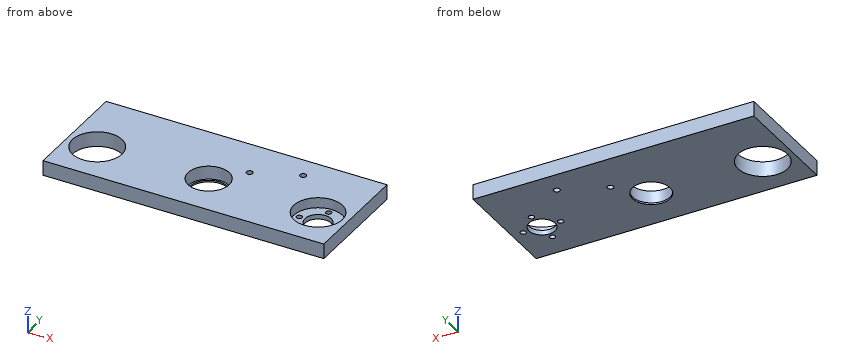
from build123d import *

# Parameters (mm, degrees)
ESQUISSE1_W                  = 150
ESQUISSE1_H                  = 60
BOSS_EXTRU_1_DEPTH           = 8
ENL_V_MAT_EXTRU_1_DEPTH      = 162.752897965
ENL_V_MAT_EXTRU_1_DEPTH_BACK = 7.1
ESQUISSE2_R                  = 11
ESQUISSE3_R                  = 10
ENL_V_MAT_EXTRU_2_DEPTH      = 162.710883987
ESQUISSE4_R                  = 7
ENL_V_MAT_EXTRU_3_DEPTH      = 162.752897965
ESQUISSE5_R                  = 13
ENL_V_MAT_EXTRU_4_DEPTH      = 5.5
ENL_V_MAT_EXTRU_5_DEPTH      = 162.752897965
ENL_V_MAT_EXTRU_5_DEPTH_BACK = 162.752897965
ESQUISSE6_R                  = 13.25
ENL_V_MAT_EXTRU_6_DEPTH      = 162.752897965
ENL_V_MAT_EXTRU_6_DEPTH_BACK = 162.752897965
ESQUISSE7_R                  = 1.65
ENL_V_MAT_EXTRU_7_DEPTH      = 162.648538503
ENL_V_MAT_EXTRU_7_DEPTH_BACK = 162.648538503
ESQUISSE8_R                  = 1.5


with BuildPart() as part:
    # Esquisse1 → Boss.-Extru.1 (new body)
    with BuildSketch(Plane.XY):
        with Locations((75, 30)):
            Rectangle(ESQUISSE1_W, ESQUISSE1_H)
    extrude(amount=BOSS_EXTRU_1_DEPTH)

    # Esquisse2 → Enlèv. mat.-Extru.1 (cut, two sides: drawn at the far end of the back side and taken through both)
    with BuildSketch(Plane.XY.offset(8).offset(-ENL_V_MAT_EXTRU_1_DEPTH_BACK)):
        with Locations(Location((75, 24, 0), (0, 0, 180))):
            Circle(ESQUISSE2_R)
    extrude(amount=ENL_V_MAT_EXTRU_1_DEPTH + ENL_V_MAT_EXTRU_1_DEPTH_BACK, mode=Mode.SUBTRACT)

    # Esquisse3 → Enlèv. mat.-Extru.2 (cut, through all)
    with BuildSketch(Plane.XY.offset(0.9)):
        with Locations((75, 24)):
            Circle(ESQUISSE3_R)
    extrude(amount=-ENL_V_MAT_EXTRU_2_DEPTH, mode=Mode.SUBTRACT)

    # Esquisse4 → Enlèv. mat.-Extru.3 (cut, through all)
    with BuildSketch(Plane.XY.offset(8)):
        with Locations((133.991524815, 23)):
            Circle(ESQUISSE4_R)
    extrude(amount=-ENL_V_MAT_EXTRU_3_DEPTH, mode=Mode.SUBTRACT)

    # Esquisse5 → Enlèv. mat.-Extru.4 (cut)
    with BuildSketch(Plane.XY.offset(8)):
        with Locations((133.991524815, 23)):
            Circle(ESQUISSE5_R)
    extrude(amount=-ENL_V_MAT_EXTRU_4_DEPTH, mode=Mode.SUBTRACT)

    # Esquisse6 → Enlèv. mat.-Extru.5 (cut, two sides: drawn at the far end of the back side and taken through both)
    with BuildSketch(Plane.XY.offset(8).offset(-ENL_V_MAT_EXTRU_5_DEPTH_BACK)):
        with Locations((16.008475185, 23)):
            Circle(ESQUISSE6_R)
    extrude(amount=ENL_V_MAT_EXTRU_5_DEPTH + ENL_V_MAT_EXTRU_5_DEPTH_BACK, mode=Mode.SUBTRACT)

    # Esquisse7 → Enlèv. mat.-Extru.6 (cut, two sides: drawn at the far end of the back side and taken through both)
    with BuildSketch(Plane.XY.offset(8).offset(-ENL_V_MAT_EXTRU_6_DEPTH_BACK)):
        with Locations((89, 38)):
            Circle(ESQUISSE7_R)
        with Locations((112, 48)):
            Circle(ESQUISSE7_R)
    extrude(amount=ENL_V_MAT_EXTRU_6_DEPTH + ENL_V_MAT_EXTRU_6_DEPTH_BACK, mode=Mode.SUBTRACT)

    # Esquisse8 → Enlèv. mat.-Extru.7 (cut, two sides: drawn at the far end of the back side and taken through both)
    with BuildSketch(Plane.XY.offset(2.5).offset(-ENL_V_MAT_EXTRU_7_DEPTH_BACK)):
        with Locations((133.991524815, 13)):
            Circle(ESQUISSE8_R)
        with Locations((123.991524815, 23)):
            Circle(ESQUISSE8_R)
        with Locations((133.991524815, 33)):
            Circle(ESQUISSE8_R)
        with Locations((143.991524815, 23)):
            Circle(ESQUISSE8_R)
    extrude(amount=ENL_V_MAT_EXTRU_7_DEPTH + ENL_V_MAT_EXTRU_7_DEPTH_BACK, mode=Mode.SUBTRACT)


solid = part.part
CAD build for the part. Positions are in the model's coordinates, mm. Round coordinates to 2 decimals unless told otherwise and drop trailing zeros. Loops run counter-clockwise (first coordinate to the right, second up) from the corner with the lowest first, then second, coordinate; pieces in that order, holes last. Notation, with made-up numbers: (-17, 58.25) - (0, 58.25) arc R32 cw to (0, 96.25) - close; hole circle Ø8 at (38.5, 23.5). An arc over 180 degrees is marked (long way). Put each result on its own line as item: value.
1. Slice it at C-C on z = 6.5. List the corners of the cut face in (x, y), and give its area (3 significant figures).
Geometry check:
outline: (0, 0) - (150, 0) - (150, 60) - (0, 60) - close; hole circle Ø26.5 at (16.01, 23); hole circle Ø22 at (75, 24); hole circle Ø3.3 at (89, 38); hole circle Ø3.3 at (112, 48); hole circle Ø26 at (133.99, 23)
area: 7,520 mm²
2. Pin check, flat tips, straight feed: P1, Ø18, axis at x = 75, y = 24, coming from the -Z side; P2, Ø23.5, axis at x = 133.99, y = 23, coming from the +Z side. Stop position of each tip, or through.
Geometry check:
P1: through
P2: z = 2.5
3. Slice it at A-A on x = 75. List the corners of the cut face in (y, z), and give its area (3 significant figures).
Geometry check:
outline: (0, 0) - (14, 0) - (14, 0.9) - (13, 0.9) - (13, 8) - (0, 8) - close; (34, 0) - (60, 0) - (60, 8) - (35, 8) - (35, 0.9) - (34, 0.9) - close
area: 306 mm²
4. Wall check: line 1 (Y direction, x = 75, z = 0.45); line 2 (Y direction, x = 18.5, z = 7); line 3 (X direction, y = 38, z = 2.75). Give the ranges that are in metal, low to high.
Geometry check:
line 1: 0 to 14, 34 to 60
line 2: 0 to 9.99, 36.01 to 60
line 3: 0 to 87.35, 90.65 to 150
5. Slice it at B-B on y = 48. List the corners of the cut face in (x, z).
Geometry check:
outline: (0, 0) - (110.35, 0) - (110.35, 8) - (0, 8) - close; (113.65, 0) - (150, 0) - (150, 8) - (113.65, 8) - close
